Verification items for the finished model (mm, model axes). A direction names the side the tool comes from. Give positions to 0.01 mm unless a question says otherwise; leave off trailing zeros. Order: outer loops, then holes, each group sorted by start corner. A loop starts at its lowest first (then second) coordinate and runs counter-clockwise, first axis right, second up. Notation, with made-up numbers: (31.5, 84) -> (55.5, 84) arc R13 ccw to (55.5, 106) -> close; hole circle Ø10 at (45.5, 37.25). An arc over 180 degrees is marked (long way). Write each question's results on one line, items separated by ' | '. Start each with the question number.
1. Mould release check, pull along Y, two halves, no side actions. Record for faces 4 (the face through (-25, -38.1, 27)), 5 (the face through (26.6, -0.5, 25.8)), 6 (the face through (-17.6, -21.1, 20.7)): +Y half, -Y half, draft (parallel to the pull), parting line (faces both ways), or undercut.
2. Cross-section at B-B, the plane y = -11. Enter the section's corners in (x, z).
3. Material ranges on L1, parallel to Z at x = 2, y = 19; L2, parallel to Y at x = 0, z = 50.5; L3, parallel to Y at x = 33, z = 5, recorded low to high. Write a range as from..to.
4. Cross-section at C-C, the plane x = -8.5. Enter the section's corners in (y, z), then the cut area to 3 significant figures.
5. Cross-section at A-A, the plane z = 26.5. Enter the section's corners in (x, y).
6. Depth check by flat-ended pin: pin 1 Ø6 at (x, y) = (-50.5, -9.5) entering from -Z; pin 2 Ø10.5 at (x, y) = (-20, -1) entering from +Z; pin 3 Ø11 at (y, z) = (-31.5, 13.5) entering from +X; pin 4 Ø4.5 at (y, z) = (-18, 6.5) entering from -X. Enter the tip coordinate at first touch or a pass-through.
7. Cross-section at D-D, the plane x = 19. Enter the section's corners in (y, z), then the cut area to 4 significant figures.
8. Set-up check for faces 1 (the face through (-30.413, -1, 4)), 2 (the face through (30, -27.976, 14)), 3 (the face through (-32, -6.568, 51)): record each of +Z, -Z, +X, -X, +Y, -Y from which the full face is reachable in a straight line by a thin tool's end or side.
from build123d import *

# Parameters (mm, degrees)
F1_DEPTH      = 38.1
F1_DEPTH_BACK = 38.1
F2_W          = 13.1363468245
F2_H          = 6.9251358509
F2_R          = 3.615061925
F3_DEPTH      = 117.9425173829
F4_W          = 35.5246793479
F4_H          = 10.1240347087
F5_DEPTH      = 52.4035820196


with BuildPart() as f1:
    # F0 (on Front) → F1 (new body, two sides)
    with BuildSketch(Plane.XZ) as f1_sk:
        Polygon((-65.5389353633, 52.4025820196), (-65.5389353633, 8.6385719478), (-30.4134916514, 8.6385719478), (-30.4134916514, 0), (52.4025820196, 0), (0, 52.4025820196), align=None)
    extrude(amount=F1_DEPTH)
    extrude(f1_sk.sketch, amount=-F1_DEPTH_BACK)

    # F2 (on face) → F3 (cut, through all)
    with BuildSketch(Plane(origin=(-65.5389353633, 0, 0), x_dir=(0, -1, 0), z_dir=(-1, 0, 0))):
        with Locations((0, 52.4025820196)):
            Rectangle(F2_W, F2_H)
        with Locations((-21.8463074416, 40.0872603059)):
            Circle(F2_R)
        with Locations((-21.8463074416, 24.2379792035)):
            Circle(F2_R)
        with Locations((21.8463074416, 24.2379792035)):
            Circle(F2_R)
        with Locations((21.8463074416, 40.0872603059)):
            Circle(F2_R)
    extrude(amount=-F3_DEPTH, mode=Mode.SUBTRACT)

    # F4 (on face) → F5 (cut, through all)
    with BuildSketch(Plane(origin=(0, 0, 0), x_dir=(1, 0, 0), z_dir=(0, 0, -1))):
        with Locations((34.6402423456, 33.0379826456)):
            Rectangle(F4_W, F4_H)
    extrude(amount=-F5_DEPTH, mode=Mode.SUBTRACT)


solid = f1.part
Results below:
1) face 4: -Y half | face 5: draft | face 6: undercut
2) outline: (-65.54, 8.64) -> (-30.41, 8.64) -> (-30.41, 0) -> (52.4, 0) -> (0, 52.4) -> (-65.54, 52.4) -> close
3) L1: z = 0..22.01, 26.47..37.86, 42.32..50.4 | L2: y = -38.1..-6.57, 6.57..38.1 | L3: y = -27.98..38.1
4) outline: (-38.1, 0) -> (38.1, 0) -> (38.1, 52.4) -> (6.57, 52.4) -> (6.57, 48.94) -> (-6.57, 48.94) -> (-6.57, 52.4) -> (-38.1, 52.4) -> close; hole circle Ø7.23 at (-21.85, 24.24); hole circle Ø7.23 at (-21.85, 40.09); hole circle Ø7.23 at (21.85, 24.24); hole circle Ø7.23 at (21.85, 40.09) | area: 3,780 mm²
5) outline: (-65.54, -38.1) -> (16.88, -38.1) -> (16.88, -27.98) -> (25.9, -27.98) -> (25.9, -24.67) -> (-65.54, -24.67) -> close; (-65.54, -19.03) -> (25.9, -19.03) -> (25.9, 19.03) -> (-65.54, 19.03) -> close; (-65.54, 24.67) -> (25.9, 24.67) -> (25.9, 38.1) -> (-65.54, 38.1) -> close
6) pin 1: stops at z = 8.64 | pin 2: stops at z = 48.94 | pin 3: stops at x = 43.13 | pin 4: stops at x = -65.54
7) outline: (-27.98, 0) -> (38.1, 0) -> (38.1, 33.4) -> (-27.98, 33.4) -> close; hole circle Ø7.23 at (-21.85, 24.24); hole circle Ø7.23 at (21.85, 24.24) | area: 2,125 mm²
8) face 1: -Z, -X, +Y, -Y | face 2: +Z, -Z, +X, -Y | face 3: +Z, +X, -X
